```python
from build123d import *

# Parameters (mm, degrees)
BOSS_EXTRUDE1_DEPTH = 3.175
SKETCH2_R           = 1.016
SKETCH2_R_2         = 1.778
CUT_EXTRUDE1_DEPTH  = 4.175


with BuildPart() as part:
    # Sketch1 → Boss-Extrude1 (new body)
    with BuildSketch(Plane.XY):
        Polygon((14.202193653, 7.22569581), (20.522953668, 1.825587343), (23.031425106, -2.643692959), (20.033036873, -4.776381895), (8.666728722, -1.668226656), (-17.619055751, -4.527501407), (-22.225, -2.643692959), (-22.225, 0), (-19.700320896, 1.210279341), (0, 5.715), (11.391452648, 8.319795747), align=None)
    extrude(amount=BOSS_EXTRUDE1_DEPTH)

    # Sketch2 → Cut-Extrude1 (cut, through all)
    with BuildSketch(Plane.XY.offset(3.175)):
        with Locations((11.153208162, 0.17748796)):
            Circle(SKETCH2_R)
        with Locations((16.551157276, -1.699576334)):
            Circle(SKETCH2_R)
        with Locations((4.951564402, 2.334026271)):
            Circle(SKETCH2_R_2)
    extrude(amount=-CUT_EXTRUDE1_DEPTH, mode=Mode.SUBTRACT)


solid = part.part
```
Geometry: final body of the model. Coordinates: model frame, mm. A direction names the side the tool comes from. Round coordinates to 2 decimals unless told otherwise and drop trailing zeros. Write each loop counter-clockwise with the first axis right and the second up, starting at its lowest first coordinate (ties: lowest second). Pieces come first, ordered by that corner, then holes. Notation, with made-up numbers: M 51.5,45 L 97.5,45 A22 cw 97.5,57 Z; hole C 10.25,24.25 d2. An arc over 180 degrees is marked long. Answer in a Markdown table with one row per item. Add a question column.
(1) Draft query along X for faces 1 (the face through (-19.89, -3.6, 1.57)), 2 (the face through (21.553, -3.695, 1.565)), 3 (the face through (-4.292, -3.078, 1.565)). Return one class per face: pulls with the +X half, pulls with the -X half, needs draft (parallel to the pull), parting line crosses it, or undercut.
(2) Cut plane C-C, the plane x = -13. Return the cut outline in (y, z) (3 decimals).
(3) Ray query, L1, parallel to Y at x = 11.5, z = 2.45; L2, parallel to Y at x = 12, z = 2.3; L3, parallel to Y at x = 8.5, z = 1.55. Return the intervals inside material, ascending.
(4) Contact query for a flat-ended pin moving along its axis: pin 1 (2.5 mm diameter, centred on x = 16.55, y = -1.7, fed in from +Z) (3 decimals). Output: stop coordinate, or through.
(5) Cut plane A-A, the plane y = 3.5. Return the cut outline in (x, z) (3 decimals), then the cut area to 3 significant figures.
(6) Cut plane D-D, the plane x = 19. Return the cut outline in (y, z) (3 decimals).
(7) Cut plane B-B, the plane z = 1.3. Return the cut outline in (x, y) (1 decimal), then the cut area to 3 significant figures.
(8) Reachability of faces 4 (the face through (17.52, -1.39, 1.61)), 5 (the face through (14.429, -3.244, 1.565)) from +Z, -Z, +X, -X, +Y, -Y: full face, straight path, thin tool, end or side. Return the list, or none.
Established:
| question | item | result |
|---|---|---|
| 1 | face 1 | pulls with the -X half |
| 1 | face 2 | pulls with the +X half |
| 1 | face 3 | undercut |
| 2 | outline | M -4.025,0 L 2.742,0 L 2.742,3.175 L -4.025,3.175 Z |
| 3 | L1 | -2.44 to -0.78, 1.13 to 8.28 |
| 3 | L2 | -2.58 to -0.38, 0.74 to 8.08 |
| 3 | L3 | -1.69 to 7.66 |
| 4 | pin 1 | z = 3.175 |
| 5 | outline | M -9.687,0 L 3.609,0 L 3.609,3.175 L -9.687,3.175 Z; M 6.294,0 L 18.563,0 L 18.563,3.175 L 6.294,3.175 Z |
| 5 | area | 81.2 mm² |
| 6 | outline | M -4.494,0 L 3.127,0 L 3.127,3.175 L -4.494,3.175 Z |
| 7 | outline | M -22.2,-2.6 L -17.6,-4.5 L 8.7,-1.7 L 20,-4.8 L 23,-2.6 L 20.5,1.8 L 14.2,7.2 L 11.4,8.3 L -19.7,1.2 L -22.2,0 Z; hole C 5,2.3 d3.6; hole C 11.2,0.2 d2; hole C 16.6,-1.7 d2 |
| 7 | area | 328 mm² |
| 8 | face 4 | +Z, -Z |
| 8 | face 5 | +Z, -Z, -Y |
